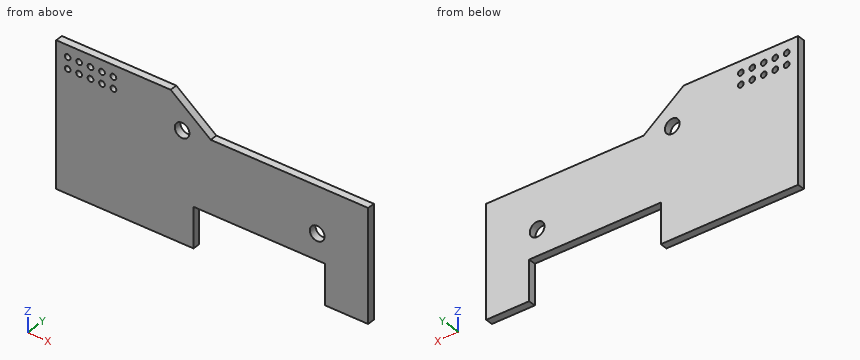
from build123d import *

# Parameters (mm, degrees)
BOSS_EXTRUDE1_DEPTH   = 1.651
SKETCH5_R             = 0.635
CUT_EXTRUDE2_DEPTH    = 2.651
F_4_CLEARANCE_HOLE1_D = 3.2639


with BuildPart() as part:
    # Sketch1 → Boss-Extrude1 (new body)
    with BuildSketch(Plane(origin=(0, 0, 0), x_dir=(1, 0, 0), z_dir=(0, 1, 0))):
        Polygon((0, 0), (30.48, 0), (30.48, -8.89), (45.085, -8.89), (59.69, -8.89), (59.69, 0), (69.215, 0), (69.215, -24.765), (45.085, -24.765), (34.29, -24.765), (25.4, -31.75), (0, -31.75), align=None)
    extrude(amount=BOSS_EXTRUDE1_DEPTH)

    # Sketch5 → Cut-Extrude2 (cut, through all)
    with BuildSketch(Plane(origin=(0, 1.651, 0), x_dir=(1, 0, 0), z_dir=(0, 1, 0))):
        with Locations(Location((2.54, -29.21, 0), (0, 0, 270))):  # turned: the seam where the file's is
            Circle(SKETCH5_R)
        with Locations(Location((5.08, -29.21, 0), (0, 0, 270))):  # turned: the seam where the file's is
            Circle(SKETCH5_R)
        with Locations(Location((7.62, -29.21, 0), (0, 0, 270))):  # turned: the seam where the file's is
            Circle(SKETCH5_R)
        with Locations(Location((10.16, -29.21, 0), (0, 0, 270))):  # turned: the seam where the file's is
            Circle(SKETCH5_R)
        with Locations(Location((12.7, -29.21, 0), (0, 0, 270))):  # turned: the seam where the file's is
            Circle(SKETCH5_R)
        with Locations(Location((2.54, -26.67, 0), (0, 0, 270))):  # turned: the seam where the file's is
            Circle(SKETCH5_R)
        with Locations(Location((5.08, -26.67, 0), (0, 0, 270))):  # turned: the seam where the file's is
            Circle(SKETCH5_R)
        with Locations(Location((7.62, -26.67, 0), (0, 0, 270))):  # turned: the seam where the file's is
            Circle(SKETCH5_R)
        with Locations(Location((10.16, -26.67, 0), (0, 0, 270))):  # turned: the seam where the file's is
            Circle(SKETCH5_R)
        with Locations(Location((12.7, -26.67, 0), (0, 0, 270))):  # turned: the seam where the file's is
            Circle(SKETCH5_R)
    extrude(amount=-CUT_EXTRUDE2_DEPTH, mode=Mode.SUBTRACT)

    # #4 Clearance Hole1 (through all)
    with Locations(Plane(origin=(0, 1.651, 0), x_dir=(-1, 0, 0), z_dir=(0, 1, 0))):
        with Locations((-27.94, 24.13), (-57.912, 14.605)):
            Hole(F_4_CLEARANCE_HOLE1_D / 2)


solid = part.part
The model under review builds one solid part; all positions refer to its coordinate system, in mm. Round coordinates to 2 decimals unless told otherwise and drop trailing zeros. Order: outer loops, then holes, each group sorted by start corner. A loop starts at its lowest first (then second) coordinate and runs counter-clockwise, first axis right, second up. Notation, with made-up numbers: (-5.5, 70) -> (12.5, 70) arc R15 cw to (12.5, 82) -> close; hole circle Ø4 at (5.25, 20). An arc over 180 degrees is marked (long way). Use CSV: the item, a comma, the result in double quotes. Start each with the question number.
(1) Consider section B-B on z = 26.67. Write out the cut boundary in (x, y) (3 decimals).
(2) Wall thickness on probe 1 along X at (y, z) = (0.65, 26.67) (3 decimals); probe 2 along Z at (x, y) = (58, 1.55) (3 decimals); probe 3 along X at (y, z) = (0.3, 4.5) (3 decimals): over which ranges is each line inside the solid? List them lowest first. Write a range as from..to.
(3) Consider section D-D on y = 0.9. State how many separate pieces and enclosed holes the cut face has, and give its area (3 significant figures).
(4) Consider section A-A on x = 10.16. Write out the cut boundary in (y, z) (3 decimals).
(5) Insertion check: pin 1 (1.1 mm diameter, centred on x = 10.16, z = 26.67, fed in from +Y); pin 2 (0.5 mm diameter, centred on x = 39, y = 0.5, fed in from -Z); pin 3 (0.8 mm diameter, centred on x = 48.5, y = 1, fed in from +Z) (3 decimals). Each pin has a flat end and moves straight along its axis. Give the tip position at first contact, or say it passes through.
(6) Consider section C-C on x = 27.94. Write out the cut boundary in (y, z), and give its area (3 significant figures).
Responses:
1,outline,"(0, 0) -> (1.905, 0) -> (1.905, 1.651) -> (0, 1.651) -> close; (3.175, 0) -> (4.445, 0) -> (4.445, 1.651) -> (3.175, 1.651) -> close; (5.715, 0) -> (6.985, 0) -> (6.985, 1.651) -> (5.715, 1.651) -> close; (8.255, 0) -> (9.525, 0) -> (9.525, 1.651) -> (8.255, 1.651) -> close; (10.795, 0) -> (12.065, 0) -> (12.065, 1.651) -> (10.795, 1.651) -> close; (13.335, 0) -> (31.865, 0) -> (31.865, 1.651) -> (13.335, 1.651) -> close"
2,probe 1,"0..1.905, 3.175..4.445, 5.715..6.985, 8.255..9.525, 10.795..12.065, 13.335..31.865"
2,probe 2,"8.89..12.975, 16.235..24.765"
2,probe 3,"0..30.48, 59.69..69.215"
3,separate pieces,"1"
3,enclosed holes,"12"
3,area,"1,630 mm²"
4,outline,"(0, 0) -> (1.651, 0) -> (1.651, 26.035) -> (0, 26.035) -> close; (0, 27.305) -> (1.651, 27.305) -> (1.651, 28.575) -> (0, 28.575) -> close; (0, 29.845) -> (1.651, 29.845) -> (1.651, 31.75) -> (0, 31.75) -> close"
5,pin 1,"through"
5,pin 2,"z = 8.89"
5,pin 3,"z = 24.765"
6,outline,"(0, 0) -> (1.65, 0) -> (1.65, 22.5) -> (0, 22.5) -> close; (0, 25.76) -> (1.65, 25.76) -> (1.65, 29.75) -> (0, 29.75) -> close"
6,area,"43.7 mm²"
